Input: part model. Units: mm. Frame: model coordinates. A direction names the side the tool comes from. Give positions to 0.01 mm unless a question says otherwise; leave off trailing zeros. Loops run counter-clockwise (first coordinate to the right, second up) from the corner with the lowest first, then second, coordinate; pieces in that order, holes last. Notation, with made-up numbers: (51, 24) - (55, 24) arc R14 cw to (55, 41) - close; hole circle Ø9 at (25, -2.75). An arc over 180 degrees is marked (long way). One line per item, written item: value.
Autodesk Inventor part; units mm, degrees
ref_plane "YZ Plane" through (0, 0, 0) normal (1, 0, 0) x (0, 1, 0)
ref_plane "XZ Plane" through (0, 0, 0) normal (0, 1, 0) x (-1, 0, 0)
sketch "Sketch1" plane through (0, 0, 0) normal (0, 0, 1) x (1, 0, 0)
  circle A0 centre (0, 0) radius 6.35
  dimension "d0" = 12.7
extrude "Extrusion1" add sketch "Sketch1" along normal mid plane 139.7
ref_plane "Work Plane1" through (0, 0, 63.5) normal (0, 0, 1) x (1, 0, 0)
sketch "Sketch2" plane through (0, 0, 63.5) normal (0, 0, 1) x (1, 0, 0)
  circle A0 centre (0, 0) radius 6.35
  circle A1 centre (0, 0) radius 6.35
  circle A2 centre (0, 0) radius 5.9436
  dimension "d4" = 12.7
  dimension "d5" = 11.8872
extrude "Extrusion2" cut sketch "Sketch2" against normal blind 0.9906
mirror "Mirror1" about plane through (0, 0, 0) normal (0, 0, 1) of "Extrusion2"
ref_plane "Work Plane3" through (0, 0, 45.4914) normal (0, 0, 1) x (1, 0, 0)
sketch "Sketch3" plane through (0, 0, 45.4914) normal (0, 0, 1) x (1, 0, 0)
  circle A0 centre (0, 0) radius 6.35
  circle A1 centre (0, 0) radius 6.35
  circle A2 centre (0, 0) radius 5.9436
  dimension "d9" = 12.7
  dimension "d10" = 11.8872
extrude "Extrusion3" cut sketch "Sketch3" along normal blind 0.9906
mirror "Mirror2" about plane through (0, 0, 0) normal (0, 0, 1) of "Extrusion3"
ref_plane "Work Plane2" through (0, 0, -63.5) normal (0, 0, 1) x (1, 0, 0)
ref_plane "Work Plane4" through (0, 0, -45.4914) normal (0, 0, 1) x (1, 0, 0)
properties part number "Stick to Scoop .5in. Pin" material "Aluminum 6061"
Item 1: Access query for faces 1 (the face through (5.669, -1.785, 45.98)), 2 (the face through (-1.38, 6.2, -54.61)). Directions: +Z, -Z, +X, -X, +Y, -Y. A direction counts if a zero-diameter tool reaches every point of the face in a straight line with its end or side. Return the directions, or none.
Verdict:
face 1: none
face 2: +Z, -Z
Item 2: Draft query along Z for faces 3 (the face through (5.669, 1.785, 63.012)), 4 (the face through (0, 0, 69.85)), 5 (the face through (-1.38, 6.2, 54.38)). Return one class per face: pulls with the +Z half, pulls with the -Z half, needs draft (parallel to the pull), parting line crosses it, or undercut.
Verdict:
face 3: undercut
face 4: pulls with the +Z half
face 5: needs draft
Item 3: Material intervals for L1, parallel to Y at x = -5, z = -38.5; L2, parallel to X at y = -3, z = 22; L3, parallel to X at y = 2.25, z = -59.5, sorted ascending.
Verdict:
L1: y = -3.91 to 3.91
L2: x = -5.6 to 5.6
L3: x = -5.94 to 5.94
Item 4: Pin query (flat end, axial travel): P1, Ø6, axis at y = 0.5, z = -22, coming from the -X side; P2, Ø3, axis at x = 4.5, z = 39, coming from the +Y side. Return the tip coordinate at first contact, or that it passes through.
Verdict:
P1: stops at x = -6.35
P2: stops at y = 5.6
Item 5: Section A-A, the plane z = 19. Output: boundary loops of the cut face in (x, y).
Verdict:
outline: circle Ø12.7 at (0, 0)
